Could you check a few things on this model? Use its own coordinates, in mm. A direction names the side the tool comes from. Coordinates: 2 decimals unless noted, no trailing zeros. Loops run counter-clockwise (first coordinate to the right, second up) from the corner with the lowest first, then second, coordinate; pieces in that order, holes last. Notation, with made-up numbers: (17, -39) - (42, -39) arc R36 cw to (42, -3) - close; hole circle Ø1 at (28.25, 49.5). An arc over 180 degrees is marked (long way). One line per item, written item: value. Start each with the question number.
(1) On a 3-axis mill with a long thin cutter (end or side, diameter ignored), from which of +Z, -Z, +X, -X, +Y, -Y can I reach the whole of each face in a straight line? I mean faces 1 (the face through (-4, -7, -93)), 2 (the face through (-7.493, 0.33, 0.952)). Say none if no direction works.
(2) If we section it at D-D on z = -20.5: Write out the boundary of the cut face in (x, y), then the cut area to 3 significant figures.
(3) If we section it at A-A on x = 0: Write out the boundary of the cut face in (y, z) (3 decimals), then the cut area to 4 significant figures.
(4) I'm going to push flat-ended pins straight in: P1, Ø8, axis at y = -5.5, z = 27, coming from the +X side; P2, Ø1.5, axis at x = 5, z = 52, coming from the -Y side; P3, Ø12, axis at x = 0, y = 0, coming from the +Z side; P4, Ø1, axis at y = 3, z = -49, coming from the +X side. Where does each tip first touch, or does it pass through?
(5) If we mould it in two halves opening along Y, with no side actions, what happens to faces 3 (the face through (-4, -7, 93)), 4 (the face through (-2.17, -9.76, 1.3)), 5 (the face through (-7.034, -2.215, -80.325))? For each: pulls with the +Y half, pulls with the -Y half, needs draft (parallel to the pull), parting line crosses it, or undercut.
(6) If I drill on line 1 along Y through (x, z) = (0, -86.75) (3 decimals); line 2 along Y through (x, z) = (0, 33.5); line 3 along X through (y, z) = (-3.5, -78), over which ranges is the centre line in solid material (lowest first)? Write a range as from..to.
(7) If we section it at C-C on y = -3.75: Write out the boundary of the cut face in (x, z), then the cut area to 3 significant figures.
(8) If we section it at B-B on z = 77.5: Write out the boundary of the cut face in (x, y) (3 decimals).
```python
from build123d import *

# Parameters (mm, degrees)
F0_R           = 10
F1_DEPTH       = 93
F4_D           = 14.75
F4_DEPTH       = 31
F4_TIP         = 4.4313470653
F4_ON_F2_D     = 14.75
F4_ON_F2_DEPTH = 31
F4_ON_F2_TIP   = 4.4313470653
F5_R           = 7.5
F6_DEPTH       = 68


with BuildPart() as f1:
    # F0 (on Top) → F1 (new body, symmetric)
    with BuildSketch(Plane.XY):
        Circle(F0_R)
    extrude(amount=F1_DEPTH, both=True)

    # F4
    with Locations(Plane.XY.offset(93)):
        with Locations((0, 0)):
            Hole(F4_D / 2, depth=F4_DEPTH)
            with Locations((0, 0, -(F4_DEPTH + F4_TIP / 2))):  # 118° drill point
                Cone(0, F4_D / 2, F4_TIP, mode=Mode.SUBTRACT)

    # F4 on F2
    with Locations(Plane(origin=(0, 0, -93), x_dir=(1, 0, 0), z_dir=(0, 0, -1))):
        with Locations((0, 0)):
            Hole(F4_ON_F2_D / 2, depth=F4_ON_F2_DEPTH)
            with Locations((0, 0, -(F4_ON_F2_DEPTH + F4_ON_F2_TIP / 2))):  # 118° drill point
                Cone(0, F4_ON_F2_D / 2, F4_ON_F2_TIP, mode=Mode.SUBTRACT)

    # F5 (on Top) → F6 (cut, symmetric)
    with BuildSketch(Plane.XY):
        Circle(F5_R)
    extrude(amount=F6_DEPTH, both=True, mode=Mode.SUBTRACT)


solid = f1.part
```
Values:
1. face 1: -Z, +X, -X, +Y, -Y
1. face 2: none
2. outline: circle Ø20 at (0, 0); hole circle Ø15 at (0, 0)
2. area: 137 mm2
3. outline: (-10, -93) - (-7.375, -93) - (-7.375, -68) - (-7.5, -68) - (-7.5, 68) - (-7.375, 68) - (-7.375, 93) - (-10, 93) - close; (7.375, -93) - (10, -93) - (10, 93) - (7.375, 93) - (7.375, 68) - (7.5, 68) - (7.5, -68) - (7.375, -68) - close
3. area: 942.5 mm2
4. P1: stops at x = 9.89
4. P2: stops at y = -9.05
4. P3: passes through
4. P4: stops at x = 9.68
5. face 3: needs draft
5. face 4: parting line crosses it
5. face 5: undercut
6. line 1: y = -10..-7.375, 7.375..10
6. line 2: y = -10..-7.5, 7.5..10
6. line 3: x = -9.37..-6.49, 6.49..9.37
7. outline: (-9.27, -93) - (-6.35, -93) - (-6.35, -68) - (-6.5, -68) - (-6.5, 68) - (-6.35, 68) - (-6.35, 93) - (-9.27, 93) - close; (6.35, -93) - (9.27, -93) - (9.27, 93) - (6.35, 93) - (6.35, 68) - (6.5, 68) - (6.5, -68) - (6.35, -68) - close
7. area: 1,050 mm2
8. outline: circle Ø20 at (0, 0); hole circle Ø14.75 at (0, 0)
